Geometry check sheet. Reference: drawing and pictorial views, mm from the part's lowest x, y, z. A direction names the side the tool comes from. Coordinates: 2 decimals unless noted, no trailing zeros. Loops run counter-clockwise (first coordinate to the right, second up) from the corner with the lowest first, then second, coordinate; pieces in that order, holes last. Notation, with made-up numbers: (82.5, 83.5) - (89.5, 83.5) arc R22 cw to (89.5, 94.5) - close; hole circle Ø8 at (-3.75, 4). An arc over 180 degrees is marked (long way). Write each question's results on one line, items separated by ' | '. Start each with the question number.
1. Cross-section at B-B (x = 7). Record the cut outline in (y, z).
2. Thickness scan on line 1 (Z direction, x = 7.25, y = 13); line 2 (X direction, y = 16, z = 4.5); line 3 (Y direction, x = 20.25, z = 1). Record the ranges inside material, lowest first. Write a range as [from, to].
3. Tool access check on the marked faces 1 and 2. Record the directions out of +Z, -Z, +X, -X, +Y, -Y that give a thin tool (end or side, any length) a straight path to the whole face; none if there is none.
4. Draft check along Y on the marked faces 3, 4 and 5. Enter one of: released by +Y, released by -Y, zero draft, split by the parting line, or undercut.
5. Cross-section at A-A (y = 28). Record the cut outline in (x, z), and give its area (3 significant figures).
6. Cross-section at D-D (z = 3.5). Record the cut outline in (x, y).
7. Cross-section at C-C (z = 7). Record the cut outline in (x, y), and give its area (3 significant figures).
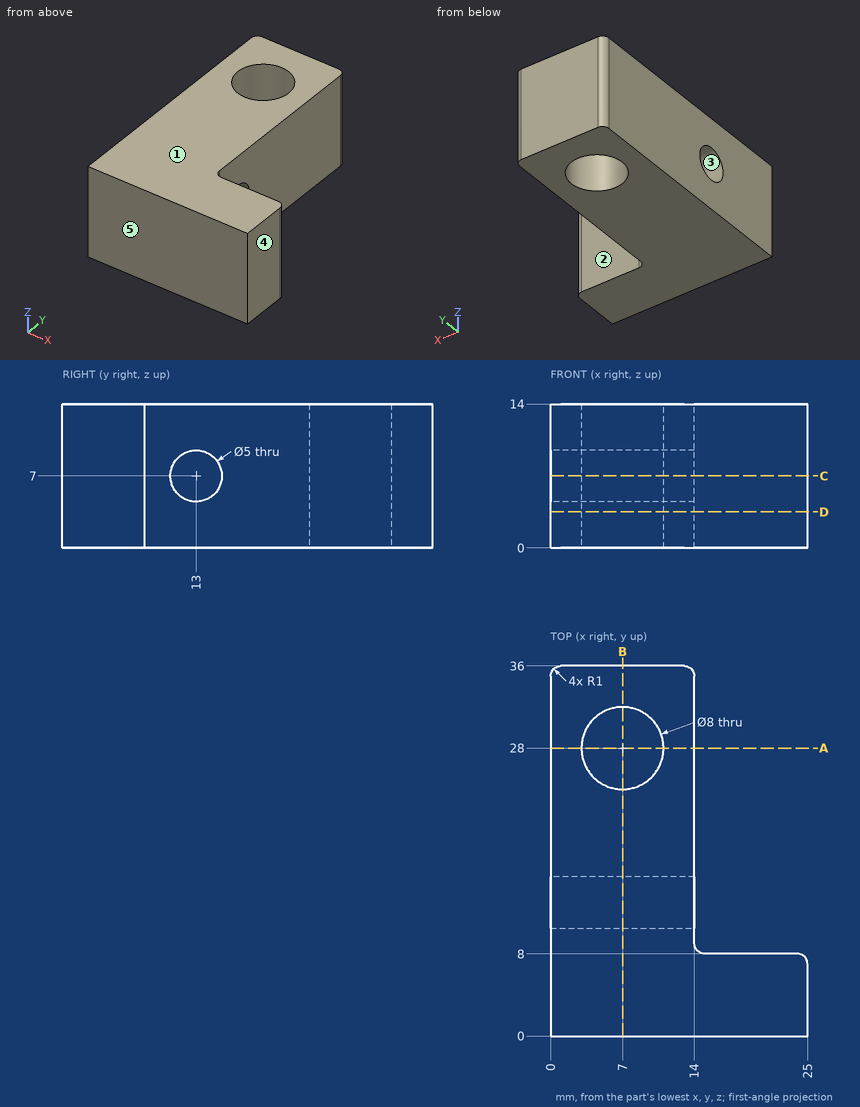
Established:
1) outline: (0, 0) - (24, 0) - (24, 14) - (0, 14) - close; (32, 0) - (36, 0) - (36, 14) - (32, 14) - close; hole circle Ø5 at (13, 7)
2) line 1: [0, 4.5], [9.5, 14] | line 2: [0, 14] | line 3: [0, 8]
3) face 1: +Z, +X, -X, +Y, -Y | face 2: +Z, -Z, +X, +Y
4) face 3: undercut | face 4: zero draft | face 5: released by -Y
5) outline: (0, 0) - (3, 0) - (3, 14) - (0, 14) - close; (11, 0) - (14, 0) - (14, 14) - (11, 14) - close | area: 84.0 mm^2
6) outline: (0, 0) - (25, 0) - (25, 7) arc R1 ccw to (24, 8) - (15, 8) arc R1 cw to (14, 9) - (14, 35) arc R1 ccw to (13, 36) - (1, 36) arc R1 ccw to (0, 35) - close; hole circle Ø8 at (7, 28)
7) outline: (0, 0) - (25, 0) - (25, 7) arc R1 ccw to (24, 8) - (15, 8) arc R1 cw to (14, 9) - (14, 10.5) - (0, 10.5) - close; (0, 15.5) - (14, 15.5) - (14, 35) arc R1 ccw to (13, 36) - (1, 36) arc R1 ccw to (0, 35) - close; hole circle Ø8 at (7, 28) | area: 471 mm^2
